Could you check a few things on this model? Use its own coordinates, in mm. A direction names the side the tool comes from. Round coordinates to 2 decimals unless told otherwise and drop trailing zeros. Order: outer loops, then holes, each group sorted by start corner. A loop starts at its lowest first (then second) coordinate and runs counter-clockwise, first axis right, second up. Notation, with made-up numbers: (86, 53) - (119, 53) arc R33 cw to (119, 92) - close; hole circle Ø4 at (50.5, -31). An arc over 180 degrees is marked (long way). Use one line per item in the form item = value.
from build123d import *

# Parameters (mm, degrees)
SKETCH1_R            = 9.415
SKETCH1_R_2          = 7.675
EXTRUDE_THIN1_DEPTH  = 10
SKETCH2_W            = 2.4
SKETCH2_H            = 11.262029822
CUT_EXTRUDE1_DEPTH   = 10
BOSS_EXTRUDE1_DEPTH  = 2
SKETCH5_R            = 1.7
CUT_EXTRUDE2_DEPTH   = 10
MOVE_START           = 3.2
MOVE_FACE1_OUTLINE_W = 10
MOVE_FACE1_OUTLINE_H = 8.338213159
MOVE_FACE1_OUTLINE_R = 1.7
MOVE_FACE1_DEPTH     = 1.2
CUT_EXTRUDE3_DEPTH   = 2.2
SKETCH8_R            = 3.25
CUT_EXTRUDE4_DEPTH   = 3


# Read off the part's stored shape, not the designer's step: Move Face1
with BuildPart() as part:
    # Sketch1 → Extrude-Thin1 (new body)
    with BuildSketch(Plane(origin=(0, 0, 0), x_dir=(1, 0, 0), z_dir=(0, 1, 0))):
        Circle(SKETCH1_R)
        Circle(SKETCH1_R_2, mode=Mode.SUBTRACT)
    extrude(amount=EXTRUDE_THIN1_DEPTH)

    # Sketch2 → Cut-Extrude1 (cut)
    with BuildSketch(Plane(origin=(0, 10, 0), x_dir=(1, 0, 0), z_dir=(0, 1, 0))):
        with Locations((0, 7.042452335)):
            Rectangle(SKETCH2_W, SKETCH2_H)
    extrude(amount=-CUT_EXTRUDE1_DEPTH, mode=Mode.SUBTRACT)

    # Sketch4 → Boss-Extrude1 (add)
    with BuildSketch(Plane(origin=(-1.2, 0, 0), x_dir=(0, 0, -1), z_dir=(1, 0, 0))):
        Polygon((9.338213159, 10), (8.459410822, 10), (8.459410822, 0), (9.338213159, 0), (15.338213159, 0), (15.338213159, 10), align=None)
    boss_extrude1 = extrude(amount=-BOSS_EXTRUDE1_DEPTH)

    # Mirror1: Boss-Extrude1 across plane
    add(boss_extrude1.mirror(Plane(origin=(0, 0, 0), x_dir=(0, 0, 1), z_dir=(1, 0, 0))))

    # Sketch5 → Cut-Extrude2 (cut)
    with BuildSketch(Plane(origin=(3.2, 0, 0), x_dir=(0, 0, -1), z_dir=(1, 0, 0))):
        with Locations((11.638213159, 5)):
            Circle(SKETCH5_R)
    extrude(amount=-CUT_EXTRUDE2_DEPTH, mode=Mode.SUBTRACT)

    # Move Face1 outline → Move Face1 (add)
    with BuildSketch(Plane.YZ.offset(MOVE_START)):
        with Locations((5, -11.169106579)):
            Rectangle(MOVE_FACE1_OUTLINE_W, MOVE_FACE1_OUTLINE_H)
        with Locations((5, -11.638213159)):
            Circle(MOVE_FACE1_OUTLINE_R, mode=Mode.SUBTRACT)
    extrude(amount=MOVE_FACE1_DEPTH)

    # Sketch7 → Cut-Extrude3 (cut)
    with BuildSketch(Plane(origin=(4.4, 0, 0), x_dir=(0, 0, -1), z_dir=(1, 0, 0))):
        Polygon((14.888213159, 5), (13.263213159, 7.814582562), (10.013213159, 7.814582562), (8.388213159, 5), (10.013213159, 2.185417438), (13.263213159, 2.185417438), align=None)
    extrude(amount=-CUT_EXTRUDE3_DEPTH, mode=Mode.SUBTRACT)

    # Sketch8 → Cut-Extrude4 (cut)
    with BuildSketch(Plane.ZY.offset(3.2)):
        with Locations((-11.638213159, 5)):
            Circle(SKETCH8_R)
    extrude(amount=CUT_EXTRUDE4_DEPTH, mode=Mode.SUBTRACT)


solid = part.part
Item 1: For faces 1 (the face through (3.315, 6.388, -14.087)), 2 (the face through (4.4, 3, -14)), 3 (the face through (1.2, 5.1, -9.7)), which set-ups out of +Z, -Z, +X, -X, +Y, -Y let a thin tool reach every point of the face, with its end or its side?
Found:
face_1 = +X
face_2 = -Z, +X, +Y, -Y
face_3 = -Z, +Y, -Y
Item 2: Will these pins go through, and if not, where does the flat tip stop? P1, Ø5.5, axis at y = 5.5, z = -12, coming from the +X side; P2, Ø0.7, axis at x = 4, z = -11, coming from the -Y side; P3, Ø8, axis at x = 0, z = -2, coming from the -Y side; P4, Ø1.7, axis at y = 6, z = -11.5, coming from the +X side.
Found:
P1 = 4.4
P2 = 0
P3 = through
P4 = 2.2
Item 3: Imagine slicing it at B-B on x = -2.75. Please give me the cut outline in (y, z).
Found:
outline = (0, -15.34) - (10, -15.34) - (10, -7.17) - (0, -7.17) - close; (0, 7.17) - (10, 7.17) - (10, 9) - (0, 9) - close; hole circle Ø3.4 at (5, -11.64)
Item 4: I need wall thicknesses on L1, parallel to X at y = 7.25, z = 0 (3 decimals); L2, parallel to Y at x = 4, z = -12.75; L3, parallel to X at y = 6.75, z = -13.5. Which ranges of each line are inside material? Lowest first, please.
Found:
L1 = -9.415 to -7.675, 7.675 to 9.415
L2 = 0 to 2.19, 7.81 to 10
L3 = -3.2 to -1.2, 1.2 to 2.2
Item 5: Imagine slicing it at A-A on z = 0. Please give me the cut outline in (x, y) (3 decimals), plus the area to 3 significant figures.
Found:
outline = (-9.415, 0) - (-7.675, 0) - (-7.675, 10) - (-9.415, 10) - close; (7.675, 0) - (9.415, 0) - (9.415, 10) - (7.675, 10) - close
area = 34.8 mm2
Item 6: If we mould it in two halves opening along Z, with no side actions, what happens to faces 4 (the face through (2.2, 6.3, -13)), 5 (the face through (-1.2, 5.1, -9.7)), 6 (the face through (-3.61, 4.98, -8.39))? For each: released by +Z, released by -Z, zero draft, split by the parting line, or undercut.
Found:
face_4 = undercut
face_5 = zero draft
face_6 = released by -Z
Item 7: Imagine slicing it at C-C on x = 5.75. Please give me the cut outline in (y, z), plus the area to 3 significant figures.
Found:
outline = (0, -7.46) - (10, -7.46) - (10, -5.08) - (0, -5.08) - close; (0, 5.08) - (10, 5.08) - (10, 7.46) - (0, 7.46) - close
area = 47.4 mm2
